Check sheet for the modelled part. Datum: model origin and axes. Units: mm. A direction names the side the tool comes from. Round coordinates to 2 decimals unless told otherwise and drop trailing zeros. Write each loop counter-clockwise with the first axis right and the second up, starting at its lowest first coordinate (ties: lowest second). Pieces come first, ordered by that corner, then holes.
from build123d import *

# Parameters (mm, degrees)
F1_DEPTH = 12.7
F3_DEPTH = 12.7
F5_DEPTH = 8.89


with BuildPart() as f1:
    # F0 (on Top) → F1 (new body)
    with BuildSketch(Plane.XY):
        with BuildLine():
            Line((0, -23.996737), (0, 0))
            Line((0, 0), (-34.743212, 0))
            Line((-34.743212, 0), (-34.743212, -23.996737))
            ThreePointArc((-34.743212, -23.996737), (-17.371606, -36.657822), (0, -23.996737))
        make_face()
    extrude(amount=F1_DEPTH)

    # F2 (on Front) → F3 (join)
    with BuildSketch(Plane.XZ):
        with BuildLine():
            Line((-34.743212, 53.041197), (-34.743212, 12.7))
            Line((-34.743212, 12.7), (0, 12.7))
            Line((0, 12.7), (0, 53.041197))
            Line((0, 53.041197), (-11.554375, 53.041197))
            Line((-11.554375, 53.041197), (-11.554375, 33.313215))
            ThreePointArc((-11.554375, 33.313215), (-17.371606, 27.495984), (-23.188837, 33.313215))
            Line((-23.188837, 33.313215), (-23.188837, 53.041197))
            Line((-23.188837, 53.041197), (-34.743212, 53.041197))
        make_face()
    extrude(amount=F3_DEPTH)

    # F4 (on face) → F5 (cut)
    with BuildSketch(Plane.YZ):
        Polygon((-18.348368, 0), (0, 0), (0, 18.348368), (-12.7, 18.348368), (-12.7, 12.7), (-18.348368, 12.7), align=None)
    extrude(amount=-F5_DEPTH, mode=Mode.SUBTRACT)


solid = f1.part
1. Set-up check for faces 1 (the flat face through (-21.5, -12.7, 28.7)), 2 (the flat face through (-8.89, -9, 9)), 3 (the flat face through (-4, -6, 18.348)): record each of +Z, -Z, +X, -X, +Y, -Y from which the full face is reachable in a straight line by a thin tool's end or side.
2. Sectioned sample at C-C, the plane y = -3.5. Enter the section's corners in (x, z).
3. Sectioned sample at D-D, the plane z = 17. Enter the section's corners in (x, y).
4. Go/stop test with flat-tipped pins: pin 1 (7 mm diameter, centred on x = -3.5, y = -5, fed in from -Z); pin 2 (3 mm diameter, centred on x = -9, y = -18.5, fed in from +Z); pin 3 (6 mm diameter, centred on x = -30, z = 36.5, fed in from -Y). Record where each tip stops, or that it passes through.
5. Sectioned sample at B-B, the plane x = -6. Enter the section's corners in (y, z).
6. Scan lines: line 1 along X through (y, z) = (-8, 45); line 2 along Z through (x, y) = (-8, -26.5); line 3 along Y through (x, z) = (-32, 16). Record each from-to range of solid material in increasing order.
7. Sectioned sample at A-A, the plane z = 45. Enter the section's corners in (x, y).
8. Release check for a two-part mould opening along X. For faces 4 (the flat face through (0, -6, 35)), 5 (the cylindrical face through (-17.693, -36.655, 6.261)), 6 (the cylindrical face through (-17.2, -6.3, 27.5)) record: released by +X, released by -X, zero draft, split by the parting line, or undercut.
Computed values:
1. face 1: +Z, +X, -X, -Y
1. face 2: -Z, +X, +Y
1. face 3: -Z, +X, +Y, -Y
2. outline: (-34.74, 0) - (-8.89, 0) - (-8.89, 18.35) - (0, 18.35) - (0, 53.04) - (-11.55, 53.04) - (-11.55, 33.31) arc R5.82 cw to (-23.19, 33.31) - (-23.19, 53.04) - (-34.74, 53.04) - close
3. outline: (-34.74, -12.7) - (-8.89, -12.7) - (-8.89, 0) - (-34.74, 0) - close
4. pin 1: stops at z = 18.35
4. pin 2: stops at z = 12.7
4. pin 3: stops at y = -12.7
5. outline: (-32.68, 0) - (-18.35, 0) - (-18.35, 12.7) - (-32.68, 12.7) - close; (-12.7, 18.35) - (0, 18.35) - (0, 53.04) - (-12.7, 53.04) - close
6. line 1: x = -34.74 to -23.19, -11.55 to 0
6. line 2: z = 0 to 12.7
6. line 3: y = -12.7 to 0
7. outline: (-34.74, -12.7) - (-23.19, -12.7) - (-23.19, 0) - (-34.74, 0) - close; (-11.55, -12.7) - (0, -12.7) - (0, 0) - (-11.55, 0) - close
8. face 4: released by +X
8. face 5: split by the parting line
8. face 6: undercut
